Here's the drawing with two shaded views (mm, measured from the low corner). I have some questions. Give positions to 0.01 mm unless a question says otherwise; leave off trailing zeros. Loops run counter-clockwise (first coordinate to the right, second up) from the corner with the lowest first, then second, coordinate; pieces in that order, holes last. Notation, with made-up numbers: M 20,30.5 L 59,30.5 A18 ccw 59,41.5 Z; hole C 60,43 d8. An arc over 180 degrees is marked long. Put each result on its own line as item: value. Start each with the question number.
1) If we mould it in two halves opening along X, with no side actions, what happens to the marked faces 1 and 2? For each: +X half, -X half, draft (parallel to the pull), parting line (faces both ways), or undercut.
2) Please list where these lines run through material, in increasing order: line 1 along Y through (x, z) = (40, 3.1); line 2 along X through (y, z) = (33, 2.95) (3 decimals); line 3 along Z through (x, y) = (34, 62). Write a range as from..to.
3) Imagine slicing it at C-C (x = 19). Write out the boundary of the cut face in (y, z), then the cut area to 3 significant figures.
4) Imagine slicing it at A-A (y = 40). Write out the boundary of the cut face in (x, z).
5) For P1, Ø3, axis at y = 24, z = 4.5, coming from the -X side; P2, Ø10, axis at x = 45.5, y = 11, coming from the +Z side; P3, Ø1, axis at y = 24, z = 1.5, coming from the +X side, each with a flat end and sliding along its axis, tell me the tip position at first contact or that it passes through.
6) Imagine slicing it at D-D (y = 71). Write out the boundary of the cut face in (x, z), then the cut area to 3 significant figures.
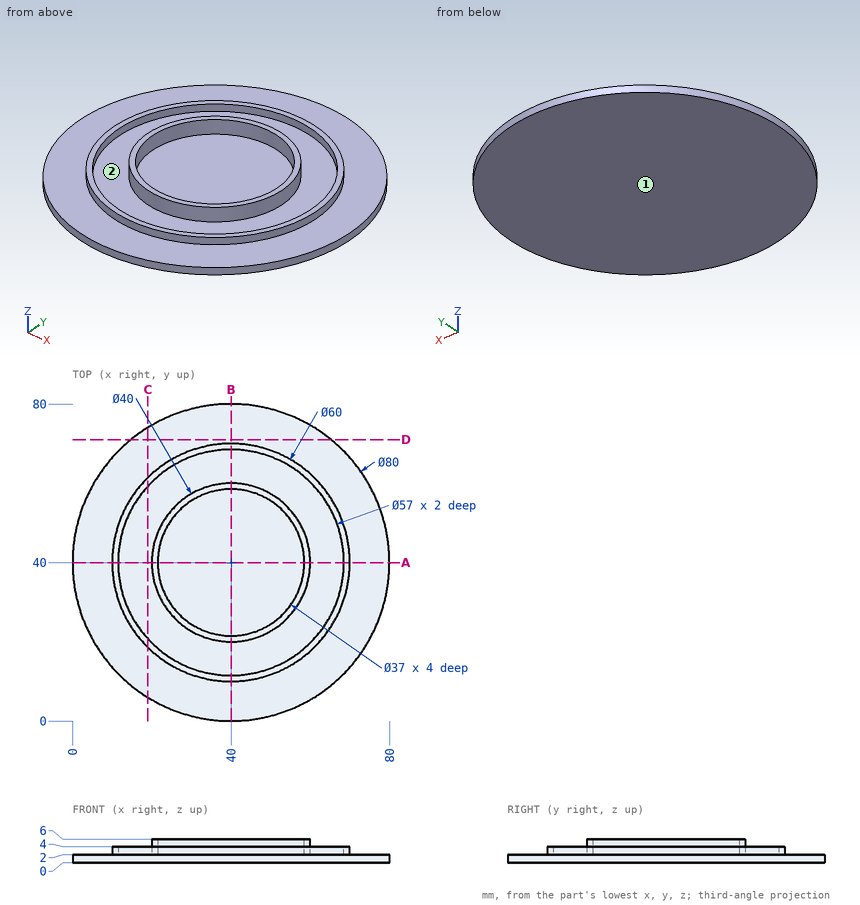
Recorded:
1. face 1: draft
1. face 2: undercut
2. line 1: 10..11.5, 20..21.5, 58.5..60, 68.5..70
2. line 2: 10.828..12.373, 21.265..22.875, 57.125..58.735, 67.627..69.172
2. line 3: 0..2
3. outline: M 5.96,0 L 74.04,0 L 74.04,2 L 61.42,2 L 61.42,4 L 59.27,4 L 59.27,2 L 20.73,2 L 20.73,4 L 18.58,4 L 18.58,2 L 5.96,2 Z
3. area: 145 mm²
4. outline: M 0,0 L 80,0 L 80,2 L 70,2 L 70,4 L 68.5,4 L 68.5,2 L 60,2 L 60,6 L 58.5,6 L 58.5,2 L 21.5,2 L 21.5,6 L 20,6 L 20,2 L 11.5,2 L 11.5,4 L 10,4 L 10,2 L 0,2 Z
5. P1: x = 13.78
5. P2: z = 4
5. P3: x = 76.87
6. outline: M 14.72,0 L 65.28,0 L 65.28,2 L 14.72,2 Z
6. area: 101 mm²
